```python
from build123d import *

# Parameters (mm, degrees)
SKETCH_1_W      = 290
SKETCH_1_H      = 195
EXTRUDE_1_DEPTH = 5
SKETCH_2_W      = 120
SKETCH_2_H      = 120
EXTRUDE_2_DEPTH = 5
FILLET_1_R      = 15
DRAFT_1_ANGLE   = 15
FILLET_2_R      = 2


with BuildPart() as part:
    # 草图1 → 凸台-拉伸1 (new body)
    with BuildSketch(Plane.XY):
        Rectangle(SKETCH_1_W, SKETCH_1_H)
    extrude(amount=EXTRUDE_1_DEPTH)

    # 草图2 → 凸台-拉伸2 (add)
    with BuildSketch(Plane.XY.offset(5)):
        with Locations((-5, 17.5)):
            Rectangle(SKETCH_2_W, SKETCH_2_H)
    extrude(amount=EXTRUDE_2_DEPTH)

    # 圆角1
    fillet_1_edges = [part.edges().sort_by_distance(p)[0] for p in [
        (-65, 77.5, 7.5),
        (-65, -42.5, 7.5),
        (55, -42.5, 7.5),
        (55, 77.5, 7.5),
    ]]
    fillet(fillet_1_edges, radius=FILLET_1_R)

    # 拔模1
    draft_1_faces = [part.faces().sort_by_distance(p)[0] for p in [
        (-65, 17.5, 7.5),
        (-60.606601718, 73.106601718, 7.5),
        (-5, 77.5, 7.5),
        (50.606601718, 73.106601718, 7.5),
        (55, 17.5, 7.5),
        (50.606601718, -38.106601718, 7.5),
        (-5, -42.5, 7.5),
        (-60.606601718, -38.106601718, 7.5),
    ]]
    draft(draft_1_faces, Plane.XY.offset(10), DRAFT_1_ANGLE)

    # 圆角2
    fillet_2_edges = [part.edges().sort_by_distance(p)[0] for p in [
        (-5, -43.839745962, 5),
        (-5, -42.5, 10),
        (-66.339745962, 17.5, 5),
        (-65, 17.5, 10),
        (55, 17.5, 10),
        (-5, 77.5, 10),
        (50.606601718, 73.106601718, 10),
        (-60.606601718, 73.106601718, 10),
        (50.606601718, -38.106601718, 10),
        (-60.606601718, -38.106601718, 10),
        (56.339745962, 17.5, 5),
        (-5, 78.839745962, 5),
        (-61.553945173, -39.053945173, 5),
        (51.553945173, -39.053945173, 5),
        (-61.553945173, 74.053945173, 5),
        (51.553945173, 74.053945173, 5),
    ]]
    fillet(fillet_2_edges, radius=FILLET_2_R)


solid = part.part
```
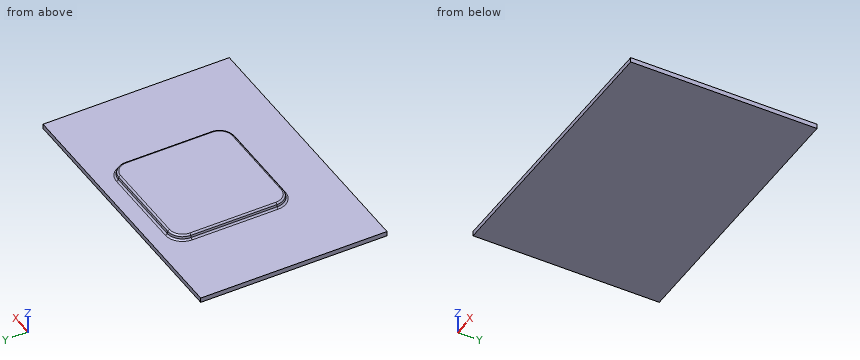
Input: part model. Units: mm. Frame: model coordinates. Round coordinates to 2 decimals unless told otherwise and drop trailing zeros. Loops run counter-clockwise (first coordinate to the right, second up) from the corner with the lowest first, then second, coordinate; pieces in that order, holes last.
1) Section query B-B on x = 36.5. Return the cut outline in (y, z), plus the area to 3 significant figures.
Ans:
outline: (-97.5, 0) - (97.5, 0) - (97.5, 5) - (80.37, 5) arc R2 cw to (78.44, 6.48) - (77.9, 8.52) arc R2 ccw to (75.97, 10) - (-40.97, 10) arc R2 ccw to (-42.9, 8.52) - (-43.44, 6.48) arc R2 cw to (-45.37, 5) - (-97.5, 5) - close
area: 1,580 mm2
2) Section query D-D on y = -73.5. Return the cut outline in (x, z), plus the area to 3 significant figures.
Ans:
outline: (-145, 0) - (145, 0) - (145, 5) - (-145, 5) - close
area: 1,450 mm2
3) Section query A-A on y = 13.5. Return the cut outline in (x, z).
Ans:
outline: (-145, 0) - (145, 0) - (145, 5) - (57.87, 5) arc R2 cw to (55.94, 6.48) - (55.4, 8.52) arc R2 ccw to (53.47, 10) - (-63.47, 10) arc R2 ccw to (-65.4, 8.52) - (-65.94, 6.48) arc R2 cw to (-67.87, 5) - (-145, 5) - close
4) Material intervals for line 1 (Z direction, x = 94.5, y = 20); line 2 (X direction, y = -31, z = 7); line 3 (Y direction, x = -10.5, z = 6), sorted ascending.
Ans:
line 1: z = 0 to 5
line 2: x = -65.41 to 55.41
line 3: y = -43.64 to 78.64
5) Section query C-C on x = -90.5. Return the cut outline in (y, z), plus the area to 3 significant figures.
Ans:
outline: (-97.5, 0) - (97.5, 0) - (97.5, 5) - (-97.5, 5) - close
area: 975 mm2
